from build123d import *

# Parameters (mm, degrees)
SKETCH1_R           = 17.5
BOSS_EXTRUDE1_DEPTH = 6


with BuildPart() as part:
    # Sketch1 → Boss-Extrude1 (new body)
    with BuildSketch(Plane(origin=(0, 0, 0), x_dir=(1, 0, 0), z_dir=(0, 1, 0))):
        with BuildLine():
            Line((50, -3), (63.416407865, -3))
            ThreePointArc((63.416407865, -3), (64.218191591, -3.402385695), (64.374722712, -4.285714286))
            ThreePointArc((64.374722712, -4.285714286), (58.227349417, -12.542357098), (48.205357143, -14.892254934))
            ThreePointArc((48.205357143, -14.892254934), (38.006177908, -16.334976641), (29.877717391, -22.662127073))
            ThreePointArc((29.877717391, -22.662127073), (0, -37.5), (-29.877717391, -22.662127073))
            ThreePointArc((-29.877717391, -22.662127073), (-38.006177908, -16.334976641), (-48.205357143, -14.892254934))
            ThreePointArc((-48.205357143, -14.892254934), (-58.227349417, -12.542357098), (-64.374722712, -4.285714286))
            ThreePointArc((-64.374722712, -4.285714286), (-64.218191591, -3.402385695), (-63.416407865, -3))
            Line((-63.416407865, -3), (-50, -3))
            ThreePointArc((-50, -3), (-47, 0), (-50, 3))
            Line((-50, 3), (-63.416407865, 3))
            ThreePointArc((-63.416407865, 3), (-64.218191591, 3.402385695), (-64.374722712, 4.285714286))
            ThreePointArc((-64.374722712, 4.285714286), (-58.227349417, 12.542357098), (-48.205357143, 14.892254934))
            ThreePointArc((-48.205357143, 14.892254934), (-38.006177908, 16.334976641), (-29.877717391, 22.662127073))
            ThreePointArc((-29.877717391, 22.662127073), (0, 37.5), (29.877717391, 22.662127073))
            ThreePointArc((29.877717391, 22.662127073), (38.006177908, 16.334976641), (48.205357143, 14.892254934))
            ThreePointArc((48.205357143, 14.892254934), (58.227349417, 12.542357098), (64.374722712, 4.285714286))
            ThreePointArc((64.374722712, 4.285714286), (64.218191591, 3.402385695), (63.416407865, 3))
            Line((63.416407865, 3), (50, 3))
            ThreePointArc((50, 3), (47, 0), (50, -3))
        make_face()
        with Locations(Location((0, 0, 0), (0, 0, 270))):
            Circle(SKETCH1_R, mode=Mode.SUBTRACT)
    extrude(amount=BOSS_EXTRUDE1_DEPTH)


solid = part.part
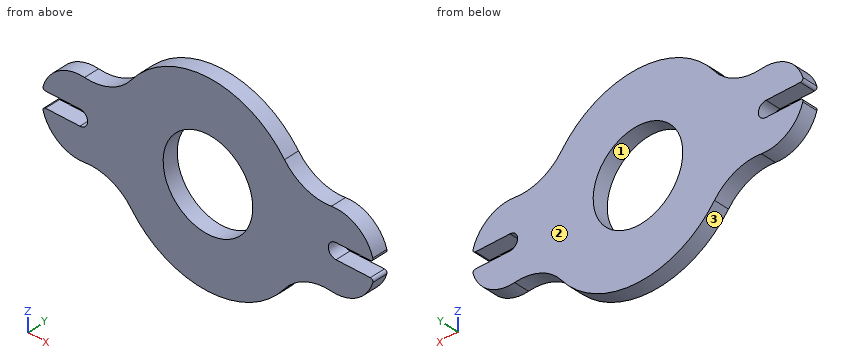
Could you check a few things on this model? Use its own coordinates, in mm. Face numbers are marked on the shaded views. Coordinates: 2 decimals unless noted, no trailing zeros. Order: outer loops, then holes, each group sorted by start corner. A loop starts at its lowest first (then second) coordinate and runs counter-clockwise, first axis right, second up.
Q1. Suppose I cut it at B-B on x = 0. Please give me the cut outline in (y, z), and give its area (3 significant figures).
Q2. Will these pins go through, and if not, where does the flat tip stop? pin 1 (1.8 mm diameter, centred on x = -55.5, y = 2.5, fed in from +Z); pin 2 (1 mm diameter, centred on x = 7.5, y = 3.5, fed in from -Z); pin 3 (2 mm diameter, centred on y = 4.5, z = -13, fed in from +X).
Q3. Please list where these lines run through material, in increasing order: L1, parallel to X at y = 2.4, z = 0; L2, parallel to X at y = 0.45, z = -12; L3, parallel to Z at x = 47.5, y = 2.75.
Q4. Suppose I cut it at D-D on x = -24.5. Please give me the cut outline in (y, z).
Q5. Thinking about a two-plate mould opening in X: for the marked faces 1, 2 and 3, which applies, released by +X, released by -X, zero draft, split by the parting line, or undercut?
Q6. Suppose I cut it at C-C on y = 4.6. Please give me the cut outline in (x, z).
Q7. Suppose I cut it at A-A on z = 0. Please give me the cut outline in (x, y).
Answer:
1. outline: (0, -37.5) - (6, -37.5) - (6, -17.5) - (0, -17.5) - close; (0, 17.5) - (6, 17.5) - (6, 37.5) - (0, 37.5) - close
1. area: 240 mm2
2. pin 1: stops at z = 14.28
2. pin 2: stops at z = -36.84
2. pin 3: stops at x = 59
3. L1: x = -47 to -17.5, 17.5 to 47
3. L2: x = -59 to -12.74, 12.74 to 59
3. L3: z = -14.82 to -1.66, 1.66 to 14.82
4. outline: (0, -28.39) - (6, -28.39) - (6, 28.39) - (0, 28.39) - close
5. face 1: undercut
5. face 2: zero draft
5. face 3: split by the parting line
6. outline: (-64.37, -4.29) arc R15 ccw to (-48.21, -14.89) arc R20 cw to (-29.88, -22.66) arc R37.5 ccw to (29.88, -22.66) arc R20 cw to (48.21, -14.89) arc R15 ccw to (64.37, -4.29) arc R1 ccw to (63.42, -3) - (50, -3) arc R3 cw to (50, 3) - (63.42, 3) arc R1 ccw to (64.37, 4.29) arc R15 ccw to (48.21, 14.89) arc R20 cw to (29.88, 22.66) arc R37.5 ccw to (-29.88, 22.66) arc R20 cw to (-48.21, 14.89) arc R15 ccw to (-64.37, 4.29) arc R1 ccw to (-63.42, 3) - (-50, 3) arc R3 cw to (-50, -3) - (-63.42, -3) arc R1 ccw to start; hole circle Ø35 at (0, 0)
7. outline: (-47, 0) - (-17.5, 0) - (-17.5, 6) - (-47, 6) - close; (17.5, 0) - (47, 0) - (47, 6) - (17.5, 6) - close
